```python
from build123d import *

# Parameters (mm, degrees)
EXTRUDE_1_DEPTH     = 5
SKETCH_2_R          = 4
EXTRUDE_2_DEPTH     = 1
SKETCH_2_3_R        = 3
CUT_EXTRUDE_1_DEPTH = 5.5
FILLET_3_R          = 0.5


with BuildPart() as part:
    # 草图1 → 凸台-拉伸1 (new body)
    with BuildSketch(Plane.XY):
        Polygon((5.773502692, 0), (2.886751346, 5), (-2.886751346, 5), (-5.773502692, 0), (-2.886751346, -5), (2.886751346, -5), align=None)
    extrude(amount=EXTRUDE_1_DEPTH)

    # 草图2 → 凸台-拉伸2 (add)
    with BuildSketch(Plane.XY.offset(5)):
        Circle(SKETCH_2_R)
    extrude(amount=EXTRUDE_2_DEPTH)

    # 草图2<3> → 切除-拉伸1 (cut, symmetric)
    with BuildSketch(Plane.XY.offset(5)):
        Circle(SKETCH_2_3_R)
    extrude(amount=CUT_EXTRUDE_1_DEPTH, both=True, mode=Mode.SUBTRACT)

    # 草图3 → 切除-旋转1 (revolve, cut)
    with BuildSketch(Plane(origin=(0, 0, 0), x_dir=(1, 0, 0), z_dir=(0, 1, 0))):
        Polygon((-5.773502692, -5), (-5.773502692, -4), (-4.773502692, -5), align=None)
    revolve(axis=Axis((0, 0, 0), (0, 0, -1)), mode=Mode.SUBTRACT)

    # 圆角3
    fillet_3_edges = [part.edges().sort_by_distance(p)[0] for p in [
        (-4, 0, 6),
    ]]
    fillet(fillet_3_edges, radius=FILLET_3_R)


solid = part.part
```
Geometry check sheet. Reference: the model listing, model coordinates, mm. A direction names the side the tool comes from. Coordinates: 2 decimals unless noted, no trailing zeros. Loops run counter-clockwise (first coordinate to the right, second up) from the corner with the lowest first, then second, coordinate; pieces in that order, holes last.
Item 1: Sectioned sample at B-B, the plane x = 0. Record the boundary of the cut face in (y, z), then the cut area to 3 significant figures.
Item 2: Sectioned sample at A-A, the plane z = 2.75. Record the boundary of the cut face in (x, y).
Item 3: Thickness scan on line 1 (Y direction, x = 0, z = 1.3); line 2 (X direction, y = -0.75, z = 2.85); line 3 (Y direction, x = 2.5, z = 3.45). Record the ranges inside material, lowest first.
Item 4: Go/stop test with flat-tipped pins: pin 1 Ø1.5 at (x, z) = (-4.5, 5) entering from +Y; pin 2 Ø3 at (x, z) = (4, 3.5) entering from -Y; pin 3 Ø2 at (y, z) = (2, 5.5) entering from -X. Record where each tip stops, or that it passes through.
Item 5: Access from +Z, -Z, +X, -X, +Y, -Y to the whole of each face (thin tool, end or side, straight path). Record for faces 1 (the face through (4.31, -2.535, 2.353)), 2 (the face through (-3, -3, 5)).
Item 6: Release check for a two-part mould opening along Y. For faces 3 (the face through (2.5, 2.3, 0)), 4 (the face through (-3, 0, 3)), 5 (the face through (4.35, 2.465, 2.353)) record: released by +Y, released by -Y, zero draft, split by the parting line, or undercut.
Check result:
1. outline: (-5, 0) - (-3, 0) - (-3, 6) - (-3.5, 6) arc R0.5 ccw to (-4, 5.5) - (-4, 5) - (-4.77, 5) - (-5, 4.77) - close; (3, 0) - (5, 0) - (5, 4.77) - (4.77, 5) - (4, 5) - (4, 5.5) arc R0.5 ccw to (3.5, 6) - (3, 6) - close
1. area: 21.8 mm2
2. outline: (-5.77, 0) - (-2.89, -5) - (2.89, -5) - (5.77, 0) - (2.89, 5) - (-2.89, 5) - close; hole circle Ø6 at (0, 0)
3. line 1: y = -5 to -3, 3 to 5
3. line 2: x = -5.34 to -2.9, 2.9 to 5.34
3. line 3: y = -5 to -1.66, 1.66 to 5
4. pin 1: stops at y = 3.37
4. pin 2: stops at y = -5
4. pin 3: stops at x = -4.91
5. face 1: +Z, -Z, +X, -Y
5. face 2: +Z
6. face 3: zero draft
6. face 4: undercut
6. face 5: released by +Y
